Can you work these out from the model? Positions are in its coordinate system, mm. A direction names the side the tool comes from. Coordinates: 2 decimals unless noted, no trailing zeros. Order: outer loops, then holes, each group sorted by start corner. A loop starts at its lowest first (then second) coordinate and runs counter-clockwise, first axis right, second up. Notation, with made-up numbers: (-37.5, 44.25) -> (12.5, 44.25) arc R16 ccw to (12.5, 48.25) -> close; hole circle Ø9 at (3, 1). An arc over 180 degrees is marked (long way). Answer in a Markdown table with one row per item.
Autodesk Inventor part; units mm, degrees
ref_plane "YZ Plane" through (0, 0, 0) normal (1, 0, 0) x (0, 1, 0)
ref_plane "XZ Plane" through (0, 0, 0) normal (0, 1, 0) x (-1, 0, 0)
ref_plane "XY Plane" through (0, 0, 0) normal (0, 0, 1) x (1, 0, 0)
sketch "Sketch1" plane through (0, 0, 0) normal (0, 1, 0) x (-1, 0, 0)
  line L0 (0, 0) -> (-90, 0)
  line L1 (-90, 0) -> (-90, -60)
  line L2 (-90, -60) -> (0, -60)
  line L3 (0, -60) -> (0, 0)
  dimension "d0" = 90
  dimension "d1" = 60
extrude "Extrusion1" add sketch "Sketch1" along normal blind 2
sketch "Sketch2" plane through (0, 2, 0) normal (0, 1, 0) x (1, 0, 0)
  line L0 (90, 0) -> (90, 60) construction
  line L1 (90, 60) -> (77.25, 60) construction
  line L2 (90, 60) -> (0, 60) construction
  line L3 (77.25, 60) -> (77.25, 0) construction
  line L4 (0, 0) -> (90, 0) construction
  line L5 (77.25, 30) -> (77.25, 35.5) construction
  line L6 (77.25, 35.5) -> (77.25, 30) construction
  line L7 (77.25, 30) -> (77.25, 24.5) construction
  line L8 (77.25, 24.5) -> (71.25, 24.5)
  line L9 (71.25, 24.5) -> (71.25, 23.5)
  line L10 (71.25, 23.5) -> (77.25, 23.5)
  line L11 (77.25, 23.5) -> (77.25, 24.5)
  line L12 (77.25, 35.5) -> (71.25, 35.5)
  line L13 (71.25, 35.5) -> (71.25, 36.5)
  line L14 (71.25, 36.5) -> (77.25, 36.5)
  line L15 (77.25, 36.5) -> (77.25, 35.5)
  dimension "d4" = 12.75
  dimension "d5" = 5.5
  dimension "d6" = 5.5
  dimension "d7" = 6
  dimension "d8" = 1
  dimension "d9" = 1
extrude "Extrusion2" cut sketch "Sketch2" against normal through all
sketch "Sketch3" plane through (0, 2, 0) normal (0, 1, 0) x (1, 0, 0)
  line L0 (77.25, 35.5) -> (71.25, 35.5) construction
  line L1 (77.25, 24.5) -> (71.25, 24.5) construction
  line L2 (71.25, 35.5) -> (71.25, 24.5) construction
  line L3 (71.25, 30) -> (64.75, 30) construction
  line L4 (64.75, 30) -> (64.75, 32.5) construction
  line L5 (64.75, 32.5) -> (59.75, 32.5) construction
  line L6 (59.75, 32.5) -> (59.75, 27.5) construction
  line L7 (59.75, 27.5) -> (64.75, 27.5) construction
  line L8 (64.75, 27.5) -> (64.75, 32.5) construction
  line L9 (59.75, 27.5) -> (62.75, 27.5) construction
  line L10 (59.75, 32.5) -> (62.75, 32.5) construction
  arc A0 (62.75, 27.5) -> (62.75, 32.5) centre (62.1875, 30) ccw
  line L11 (62.75, 32.5) -> (59.75, 32.5) construction
  line L12 (59.75, 32.5) -> (59.75, 27.5) construction
  line L13 (59.75, 32.5) -> (62.75, 32.5)
  line L14 (59.75, 32.5) -> (59.75, 27.5)
  line L15 (59.75, 27.5) -> (62.75, 27.5)
  point P0 (0, 0)
  dimension "d12" = 6.5
  dimension "d15" = 2.5
  dimension "d16" = 5
  dimension "d17" = 5
  dimension "d18" = 3
  dimension "d19" = 3
extrude "Extrusion3" cut sketch "Sketch3" against normal through all
sketch "Sketch20" plane through (0, 2, 0) normal (0, 1, 0) x (1, 0, 0)
  line L0 (77.25, 36.5) -> (77.25, 35.5) construction
  line L1 (77.25, 36.5) -> (59.75, 36.5) construction
  line L2 (59.75, 23.5) -> (77.25, 23.5) construction
  line L3 (77.25, 23.5) -> (77.25, 36.5) construction
  line L4 (68.5, 30) -> (77.25, 30) construction
  line L5 (68.5, 30) -> (68.5, 29.5) construction
  line L6 (68.5, 29.5) -> (77.25, 29.5)
  line L7 (77.25, 29.5) -> (77.25, 30.5)
  line L8 (77.25, 30.5) -> (68.5, 30.5)
  line L9 (68.5, 30.5) -> (68.5, 29.5)
  line L10 (68.933, 30.25) -> (64.558, 37.8277)
  line L11 (63.692, 37.3277) -> (68.067, 29.75)
  line L12 (68.067, 29.75) -> (68.933, 30.25)
  line L13 (69.7542, 40.8277) -> (58.4958, 34.3277) construction
  line L14 (68.067, 30.25) -> (63.692, 22.6723)
  line L15 (64.558, 22.1723) -> (68.933, 29.75)
  line L16 (68.933, 29.75) -> (68.067, 30.25)
  line L17 (58.4958, 25.6723) -> (69.7542, 19.1723) construction
  line L18 (63.692, 37.3277) -> (64.558, 37.8277)
  line L19 (63.692, 22.6723) -> (64.558, 22.1723)
  point P0 (0, 0)
  point P1 (64.125, 37.5777)
  point P2 (64.125, 22.4223)
  dimension "d143" = 13
  dimension "d144" = 0.5
  dimension "d145" = 1
  dimension "d148" = 360
extrude "Extrusion17" add sketch "Sketch20" along normal blind 10
sketch "Sketch21" plane through (0, 2, 0) normal (0, 1, 0) x (1, 0, 0)
  line L0 (77.25, 24.5) -> (77.25, 23.5) construction
  line L1 (77.25, 23.5) -> (59.75, 23.5) construction
  line L2 (59.75, 23.5) -> (59.75, 36.5) construction
  line L3 (59.75, 36.5) -> (77.25, 36.5) construction
  line L4 (77.25, 36.5) -> (77.25, 23.5) construction
  circle A0 centre (68.5, 30) radius 12.5
  circle A1 centre (68.5, 30) radius 13.5
  point P0 (0, 0)
  dimension "d154" = 13
  dimension "d155" = 25
  dimension "d156" = 27
extrude "Extrusion18" add sketch "Sketch21" along normal blind 5
sketch "Sketch23" plane through (0, 2, 0) normal (0, 1, 0) x (1, 0, 0)
  line L0 (90, 0) -> (90, 60) construction
  line L1 (90, 30) -> (87, 30) construction
  line L2 (87, 30) -> (87, 18.5) construction
  line L3 (87, 18.5) -> (50, 18.5) construction
  line L4 (50, 18.5) -> (50, 41.5) construction
  line L5 (50, 41.5) -> (87, 41.5) construction
  line L6 (87, 41.5) -> (87, 18.5) construction
  line L7 (87, 18.5) -> (87, 15.5) construction
  line L8 (87, 15.5) -> (82, 15.5) construction
  line L9 (87, 15.5) -> (82, 15.5)
  line L10 (82, 15.5) -> (82, 44.5)
  line L11 (82, 44.5) -> (87, 44.5)
  line L12 (87, 44.5) -> (87, 15.5)
  line L13 (50, 18.5) -> (50, 15.5) construction
  line L14 (50, 15.5) -> (55, 15.5)
  line L15 (55, 15.5) -> (55, 44.5)
  line L16 (55, 44.5) -> (50, 44.5)
  line L17 (50, 44.5) -> (50, 15.5)
  point P0 (0, 0)
  dimension "d164" = 3
  dimension "d165" = 11.5
  dimension "d166" = 37
  dimension "d167" = 23
  dimension "d168" = 3
  dimension "d169" = 5
  dimension "d170" = 5
  dimension "d171" = 29
  dimension "d172" = 3
  dimension "d173" = 5
  dimension "d174" = 29
extrude "Extrusion19" add sketch "Sketch23" along normal blind 5
sketch "Sketch24" plane through (0, 2, 0) normal (0, 1, 0) x (1, 0, 0)
  line L0 (84, 8.5) -> (82.5, 8.5) construction
  line L1 (82.5, 8.5) -> (8.5, 8.5) construction
  line L2 (8.5, 8.5) -> (8.5, 6.9) construction
  line L3 (8.5, 6.9) -> (82.5, 6.9) construction
  line L4 (82.5, 6.9) -> (82.5, 8.5) construction
  line L5 (82.5, 6.9) -> (77.5, 6.9)
  line L6 (77.5, 6.9) -> (77.5, 5.4)
  line L7 (77.5, 5.4) -> (84, 5.4)
  line L8 (82.5, 6.9) -> (82.5, 8.5)
  line L9 (82.5, 8.5) -> (77.5, 8.5)
  line L10 (77.5, 8.5) -> (77.5, 10)
  line L11 (8.5, 6.9) -> (13.5, 6.9)
  line L12 (13.5, 6.9) -> (13.5, 5.4)
  line L13 (13.5, 5.4) -> (7, 5.4)
  line L14 (8.5, 8.5) -> (13.5, 8.5)
  line L15 (13.5, 8.5) -> (13.5, 10)
  line L16 (13.5, 10) -> (7, 10)
  line L17 (7, 10) -> (7, 5.4)
  line L18 (8.5, 6.9) -> (8.5, 8.5)
  line L19 (77.5, 10) -> (84, 10)
  line L20 (84, 5.4) -> (84, 10)
  line L21 (84, 8.5) -> (90, 8.5) construction
  line L22 (90, 0) -> (90, 60) construction
  line L23 (87, 44.5) -> (87, 15.5) construction
  line L24 (87, 15.5) -> (90, 15.5) construction
  line L25 (90, 8.5) -> (90, 15.5) construction
  point P0 (0, 0)
  dimension "d178" = 1.5
  dimension "d179" = 74
  dimension "d180" = 1.6
  dimension "d181" = 5
  dimension "d182" = 1.5
  dimension "d183" = 5
  dimension "d184" = 1.5
  dimension "d185" = 5
  dimension "d186" = 1.5
  dimension "d187" = 6.5
  dimension "d188" = 5
  dimension "d189" = 1.5
  dimension "d230" = 6
  dimension "d231" = 7
extrude "Extrusion20" add sketch "Sketch24" along normal blind 4
sketch "Sketch25" plane through (0, 6, 0) normal (0, 1, 0) x (1, 0, 0)
  line L0 (84, 5.4) -> (84, 10)
  line L1 (77.5, 5.4) -> (84, 5.4)
  line L2 (84, 5.4) -> (84, 10)
  line L3 (84, 10) -> (77.5, 10)
  line L4 (84, 10) -> (77.5, 10)
  line L5 (77.5, 10) -> (77.5, 8.5)
  line L6 (77.5, 10) -> (77.5, 8.5)
  line L7 (77.5, 8.5) -> (82.5, 8.5)
  line L8 (77.5, 8.5) -> (82.5, 8.5)
  line L9 (82.5, 6.9) -> (82.5, 8.5)
  line L10 (82.5, 8.5) -> (82.5, 6.9)
  line L11 (82.5, 6.9) -> (77.5, 6.9)
  line L12 (77.5, 5.4) -> (77.5, 6.9)
  point P0 (0, 0)
extrude "Extrusion21" add sketch "Sketch25" along normal blind 4
sketch "Sketch26" plane through (0, 2, 0) normal (0, 1, 0) x (1, 0, 0)
  line L0 (50, 15.5) -> (55, 15.5)
  line L1 (45, 23) -> (5, 23)
  line L2 (5, 23) -> (5, 38)
  line L3 (5, 38) -> (45, 38)
  line L4 (45, 38) -> (45, 23)
  line L5 (50, 15.5) -> (50, 0) construction
  line L6 (50, 0) -> (45, 0) construction
  line L7 (0, 0) -> (90, 0) construction
  line L8 (45, 23) -> (45, 0) construction
  dimension "d195" = 40
  dimension "d196" = 15
  dimension "d229" = 23
extrude "Extrusion22" add sketch "Sketch26" along normal blind 15
sketch "Sketch27" plane through (45, 2, -38) normal (0, 0, -1) x (-1, 0, 0)
  line L0 (40, 15) -> (0, 15)
  circle A0 centre (20, 15) radius 15
  point P0 (45, -2)
  dimension "d199" = 30
extrude "Extrusion23" cut sketch "Sketch27" against normal blind 15
sketch "Sketch29" plane through (0, 2, 0) normal (0, 1, 0) x (1, 0, 0)
  line L0 (25, 38) -> (45, 38)
  line L1 (45, 38) -> (45, 46) construction
  line L2 (45, 46) -> (-7, 46) construction
  line L3 (-7, 46) -> (-7, 47.6) construction
  line L4 (-7, 47.6) -> (45, 47.6) construction
  line L5 (45, 47.6) -> (45, 46) construction
  line L6 (45, 46) -> (40, 46)
  line L7 (40, 46) -> (40, 44.5)
  line L8 (40, 44.5) -> (46.5, 44.5)
  line L9 (45, 46) -> (45, 47.6)
  line L10 (45, 47.6) -> (40, 47.6)
  line L11 (40, 47.6) -> (40, 49.1)
  line L12 (40, 49.1) -> (46.5, 49.1)
  line L13 (46.5, 49.1) -> (46.5, 44.5)
  line L14 (-7, 47.6) -> (-7, 46)
  line L15 (-7, 46) -> (-2, 46)
  line L16 (-2, 46) -> (-2, 44.5)
  line L17 (-2, 44.5) -> (-8.5, 44.5)
  line L18 (-7, 47.6) -> (-2, 47.6)
  line L19 (-2, 47.6) -> (-2, 49.1)
  line L20 (-2, 49.1) -> (-8.5, 49.1)
  line L21 (-8.5, 49.1) -> (-8.5, 44.5)
  point P0 (0, 0)
  dimension "d215" = 8
  dimension "d216" = 52
  dimension "d217" = 1.6
  dimension "d218" = 5
  dimension "d219" = 1.5
  dimension "d220" = 6.5
  dimension "d221" = 1.5
  dimension "d222" = 5
  dimension "d223" = 6.5
  dimension "d224" = 6.5
extrude "Extrusion25" add sketch "Sketch29" along normal blind 4
sketch "Sketch30" plane through (0, 0, -60) normal (-1, 0, 0) x (0, 0, 1)
  line L0 (0, 0) -> (0, 2)
  line L1 (60, 0) -> (60, 2)
  line L2 (0, 0) -> (60, 0)
  line L3 (60, 0) -> (60, 2)
  line L4 (60, 2) -> (0, 2)
  line L5 (0, 2) -> (0, 0)
extrude "Extrusion26" add sketch "Sketch30" along normal blind 10.5
sketch "Sketch31" plane through (0, 2, 0) normal (0, 1, 0) x (1, 0, 0)
  arc A0 (90, 55) -> (85, 60) centre (85, 55) ccw
  arc A1 (-10.5, 5) -> (-5.5, 0) centre (-5.5, 5) ccw
  arc A2 (-5.5, 60) -> (-10.5, 55) centre (-5.5, 55) ccw
  arc A3 (85, 0) -> (90, 5) centre (85, 5) ccw
  line L0 (90, 0) -> (85, 0)
  line L1 (90, 0) -> (90, 5)
  line L2 (-5.5, 0) -> (-10.5, 0)
  line L3 (-10.5, 55) -> (-10.5, 60)
  line L4 (-10.5, 60) -> (-5.5, 60)
  line L5 (85, 60) -> (90, 60)
  line L6 (90, 60) -> (90, 55)
  line L7 (-10.5, 0) -> (-10.5, 5)
  point P0 (0, 0)
  dimension "d232" = 5
extrude "Extrusion27" cut sketch "Sketch31" against normal through all
properties part number "base"
(1) We'd pull the mould along Z, two halves only. Please class faces 6 (the flat face through (52, 4, -15.5)), 7 (the flat face through (7, 4, -8)), 8 (the cylindrical face through (58.58, 4.465, -37.606)): +Z half, -Z half, draft (parallel to the pull), parting line (faces both ways), or undercut.
Response values:
| item | result |
|---|---|
| face 6 | +Z half |
| face 7 | draft |
| face 8 | undercut |
(2) Suppose I cut it at A-A (y = 8.75). Please give me the cut outline in (x, z).
Response values:
| item | result |
|---|---|
| outline | (5, -38) -> (12.47, -38) -> (12.47, -23) -> (5, -23) -> close; (37.53, -38) -> (45, -38) -> (45, -23) -> (37.53, -23) -> close; (63.69, -37.33) -> (64.56, -37.83) -> (68.79, -30.5) -> (77.25, -30.5) -> (77.25, -29.5) -> (68.79, -29.5) -> (64.56, -22.17) -> (63.69, -22.67) -> (67.92, -30) -> close; (77.5, -10) -> (84, -10) -> (84, -5.4) -> (77.5, -5.4) -> (77.5, -6.9) -> (82.5, -6.9) -> (82.5, -8.5) -> (77.5, -8.5) -> close |
(3) I need wall thicknesses on line 1 (Z direction, x = 66, y = 2.25); line 2 (Z direction, x = 68.5, y = 4.9); line 3 (X direction, y = 11.5, z = -35). Which ranges of each line are inside material? Lowest first, please. Write a range as [from, to].
Response values:
| item | result |
|---|---|
| line 1 | [-43.27, -42.25], [-35.33, -33.33], [-26.67, -24.67], [-17.75, -16.73] |
| line 2 | [-43.5, -42.5], [-31, -29], [-17.5, -16.5] |
| line 3 | [5, 11.04], [38.96, 45], [65.04, 66.19] |
(4) On a 3-axis mill with a long thin cutter (end or side, diameter ignored), from which of +Z, -Z, +X, -X, +Y, -Y can I reach the whole of each face in a straight line? I mean faces 1 (the flat face through (10, 4, -10)), 2 (the flat face through (45, 9, -31)), 3 (the flat face through (65.84, 6.93, -26.39)), 4 (the flat face through (46.5, 4, -47)), 5 (the flat face through (53, 4, -44.5)). Say none if no direction works.
Response values:
| item | result |
|---|---|
| face 1 | +X, -X, +Y |
| face 2 | +Z, +Y |
| face 3 | +Y |
| face 4 | +Z, -Z, +X, +Y |
| face 5 | -Z, +X, +Y |
(5) Will these pins go through, and if not, where does the flat tip stop? pin 1 Ø0.8 at (y, z) = (4.5, -8) entering from -X; pin 2 Ø6 at (y, z) = (13.5, -39) entering from -X; pin 3 Ø4.5 at (x, y) = (9, 4.5) entering from -Z.
Response values:
| item | result |
|---|---|
| pin 1 | x = 7 |
| pin 2 | x = 5 |
| pin 3 | z = -38 |
(6) Suppose I cut it at B-B (x = 12.5). Please give me the cut outline in (y, z), and give its area (3 significant figures).
Response values:
| item | result |
|---|---|
| outline | (0, -60) -> (2, -60) -> (2, -38) -> (8.71, -38) -> (8.71, -23) -> (2, -23) -> (2, -10) -> (6, -10) -> (6, -8.5) -> (2, -8.5) -> (2, -6.9) -> (6, -6.9) -> (6, -5.4) -> (2, -5.4) -> (2, 0) -> (0, 0) -> close |
| area | 233 mm2 |
(7) Suppose I cut it at D-D (x = 30.5). Please give me the cut outline in (y, z), and give its area (3 significant figures).
Response values:
| item | result |
|---|---|
| outline | (0, -60) -> (2, -60) -> (2, -38) -> (3.04, -38) -> (3.04, -23) -> (2, -23) -> (2, 0) -> (0, 0) -> close |
| area | 136 mm2 |
